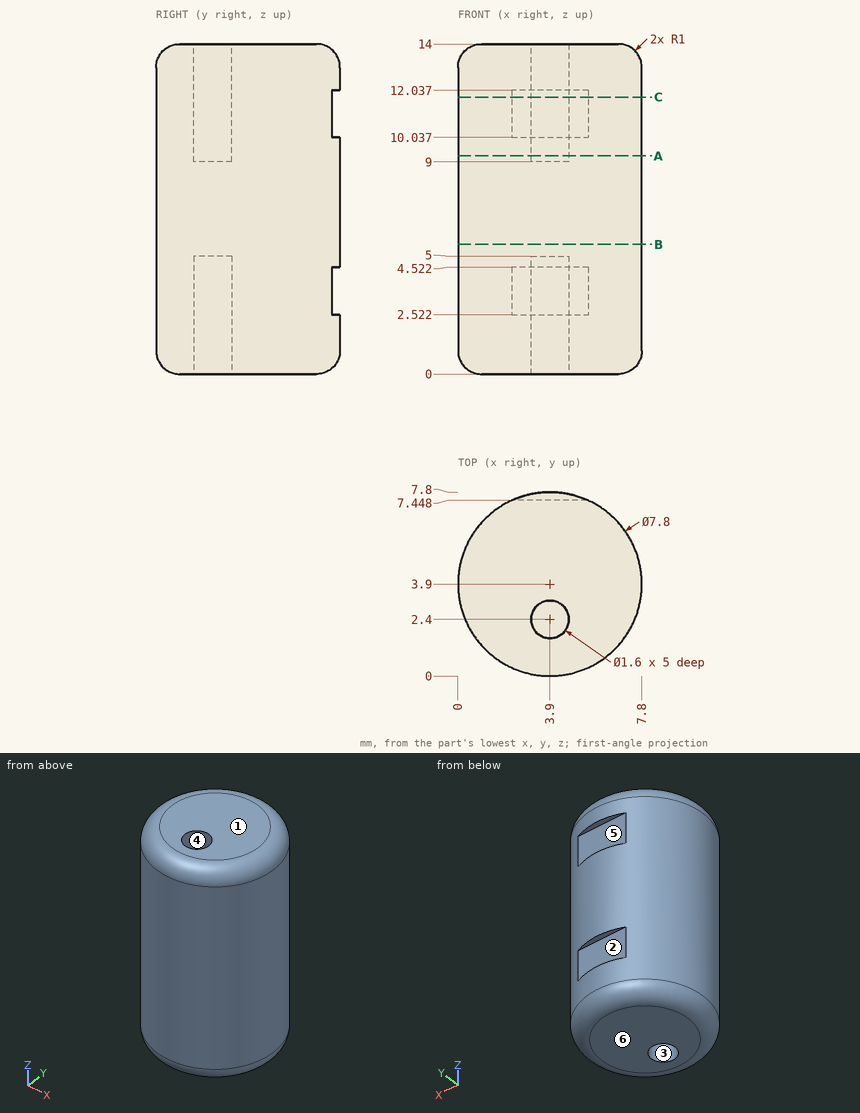
For this review, use the dimensioned drawing (mm, ordinates from the lowest corner) and the shaded views. A direction names the side the tool comes from. Coordinates: 2 decimals unless noted, no trailing zeros. Order: outer loops, then holes, each group sorted by start corner. A loop starts at its lowest first (then second) coordinate and runs counter-clockwise, first axis right, second up. Notation, with made-up numbers: M 57.5,-10.75 L 71.5,-10.75 A24 ccw 71.5,15.25 Z; hole C 58,40.25 d6. An arc over 180 degrees is marked long. Answer as a JSON object with one key per item and string values. Group by question number.
1) Tool access review of the marked faces 1, 2 and 3: name each direction out of +Z, -Z, +X, -X, +Y, -Y from which nothing blocks a thin tool from reaching the whole face with its end or side.
2) Wall thickness on L1, parallel to Y at x = 3.9, z = 2.3; L2, parallel to Y at x = 3.9, z = 11.35; L3, parallel to Y at x = 2, z = 1.5 (1 decimal): over which ranges is each line inside the solid? List them lowest first.
3) Add section A-A, the plane z = 9.25. Write out the cut boundary in (x, y).
4) For pin 1 (3 mm diameter, centred on x = 6, z = 12, fed in from +Y); pin 2 (1 mm diameter, centred on x = 6, y = 7, fed in from +Z); pin 3 (1 mm diameter, centred on x = 4, z = 11.5, fed in from +Y), all flat-tipped, find the tip position at first contact; note any pin that passes through.
5) Add section C-C, the plane z = 11.75. Write out the cut boundary in (x, y), then the cut area to 3 significant figures.
6) Mouldability with a two-part tool opening along Z and no side actions: class the marked faces 4, 5 and 6 as pulls with the +Z half, pulls with the -Z half, needs draft (parallel to the pull), parting line crosses it, or undercut.
7) Add section B-B, the plane z = 5.5. Write out the cut boundary in (x, y), then the cut area to 3 significant figures.
Computed values:
{
 "1": {"face 1": "+Z, +X, -X, +Y, -Y", "face 2": "+X, -X, +Y", "face 3": "-Z"},
 "2": {"L1": "y = 0 to 1.6, 3.2 to 7.8", "L2": "y = 0 to 1.6, 3.2 to 7.45", "L3": "y = 0.5 to 7.3"},
 "3": {"outline": "C 3.9,3.9 d7.8; hole C 3.9,2.4 d1.6"},
 "4": {"pin 1": "stops at y = 7.75", "pin 2": "stops at z = 13.94", "pin 3": "stops at y = 7.45"},
 "5": {"outline": "M 2.28,7.45 A3.9 ccw long 5.52,7.45 Z; hole C 3.9,2.4 d1.6", "area": "45.0 mm^2"},
 "6": {"face 4": "needs draft", "face 5": "undercut", "face 6": "pulls with the -Z half"},
 "7": {"outline": "C 3.9,3.9 d7.8", "area": "47.8 mm^2"}
}
